For this review, take the finished solid that the model builds, in its own axes (mm). A direction names the side the tool comes from. Round coordinates to 2 decimals unless told otherwise and drop trailing zeros. Order: outer loops, then holes, each group sorted by start corner. A loop starts at its lowest first (then second) coordinate and runs counter-clockwise, first axis right, second up. Notation, with made-up numbers: M -28.75,-26.5 L -14.75,-26.5 A19 cw -14.75,-10.5 Z; hole C -4.5,47 d3. An arc over 180 degrees is marked long. Answer as a JSON object with one key per item and string values.
Autodesk Inventor part; units mm, degrees
ref_plane "YZ Plane" through (0, 0, 0) normal (1, 0, 0) x (0, 1, 0)
ref_plane "XZ Plane" through (0, 0, 0) normal (0, 1, 0) x (-1, 0, 0)
ref_plane "XY Plane" through (0, 0, 0) normal (0, 0, 1) x (1, 0, 0)
sketch "Sketch4" plane through (0, 0, 0) normal (0, 1, 0) x (-1, 0, 0)
  line L0 (0, 0) -> (0, 66)
  line L1 (0, 66) -> (15, 66)
  line L2 (15, 66) -> (15, 50.5)
  line L3 (15, 50.5) -> (5, 50.5)
  line L4 (5, 50.5) -> (5, 46.5)
  line L5 (5, 46.5) -> (15, 46.5)
  line L6 (15, 46.5) -> (15, 0)
  line L7 (15, 0) -> (0, 0)
  dimension "d6" = 66
  dimension "d7" = 15
  dimension "d8" = 15.5
  dimension "d9" = 10
  dimension "d10" = 4
revolve "Revolution1" add sketch "Sketch4" angle 360 about axis through (-15, 0, 0) along (1, 0, 0)
sketch "Sketch5" plane through (-15, 0, 0) normal (-1, 0, 0) x (0, 0, 1)
  point P0 (0, 0)
sketch "Sketch6" plane through (-15, 0, 0) normal (-1, 0, 0) x (0, 0, 1)
  circle A0 centre (0, 0) radius 59
  point P0 (59, 0)
  point P1 (0, -59)
  point P2 (-59, 0)
  point P3 (0, 59)
  dimension "d13" = 118
hole "Hole1" at (-15, 0, 59) at (-15, -59, 0) at (-15, 0, -59) at (-15, 59, 0) direction (1, 0, 0) diameter 6.6 end through all
properties part number "100mm-FlangeBottom-Sketch"
1) Machinability: for faces 4 (the flat face through (-5, 15, 45)), 5 (the flat face through (-15, 49, 14)), which of the approach directions +Z, -Z, +X, -X, +Y, -Y give a long, thin tool a straight path to every point of the face, cutting with its end or side? Answer none if there is none.
Geometry check:
{"face 4": "-X", "face 5": "+Z, -Z, -X, +Y, -Y"}
2) Add section D-D on y = -59. State the section outline as (x, z) points, and give its area (3 significant figures).
Geometry check:
{"outline": "M -15,-29.58 L 0,-29.58 L 0,-3.3 L -15,-3.3 Z; M -15,3.3 L 0,3.3 L 0,29.58 L -15,29.58 Z", "area": "788 mm²"}
3) For L1, parallel to Y at x = -7.75, z = 0; L2, parallel to Z at x = -9.25, y = -37; L3, parallel to Y at x = -6.5, z = 11, list the stretches that pass through material, from the lowest coordinate up.
Geometry check:
{"L1": "y = -66 to -62.3, -55.7 to -50.5, -46.5 to 46.5, 50.5 to 55.7, 62.3 to 66", "L2": "z = -54.65 to -34.37, -28.16 to 28.16, 34.37 to 54.65", "L3": "y = -65.08 to -49.29, -45.18 to 45.18, 49.29 to 65.08"}
4) Mouldability with a two-part tool opening along Y and no side actions: class faces 1 (the flat face through (0, -1, -1)), 2 (the cylindrical face through (-7.4, -0.1, -62.3)), 3 (the cylindrical face through (-7.605, -25.278, 60.967)) as +Y half, -Y half, draft (parallel to the pull), parting line (faces both ways), or undercut.
Geometry check:
{"face 1": "draft", "face 2": "undercut", "face 3": "parting line"}
5) Add section A-A on x = -9.5. State the section outline as (y, z) points.
Geometry check:
{"outline": "C 0,0 d132; C 0,0 d93; hole C -59,0 d6.6; hole C 0,0 d101; hole C 0,-59 d6.6; hole C 0,59 d6.6; hole C 59,0 d6.6"}
6) Insertion check: P1, Ø5, axis at x = -8.5, y = -32.5, coming from the +Z side; P2, Ø5.5, axis at y = -59, z = 0, coming from the -X side; P3, Ø1.5, axis at x = -3, z = -40, coming from the -Y side; P4, Ø1, axis at x = -11, z = -22, coming from the +Y side. Each pin has a flat end and moves straight along its axis. Give the tip position at first contact, or say it passes through.
Geometry check:
{"P1": "stops at z = 58.79", "P2": "passes through", "P3": "stops at y = -53.06", "P4": "stops at y = 62.4"}
7) Add section B-B on z = 0. State the section outline as (x, y) points.
Geometry check:
{"outline": "M -15,-66 L 0,-66 L 0,-62.3 L -15,-62.3 Z; M -15,-55.7 L 0,-55.7 L 0,55.7 L -15,55.7 L -15,50.5 L -5,50.5 L -5,46.5 L -15,46.5 L -15,-46.5 L -5,-46.5 L -5,-50.5 L -15,-50.5 Z; M -15,62.3 L 0,62.3 L 0,66 L -15,66 Z"}
